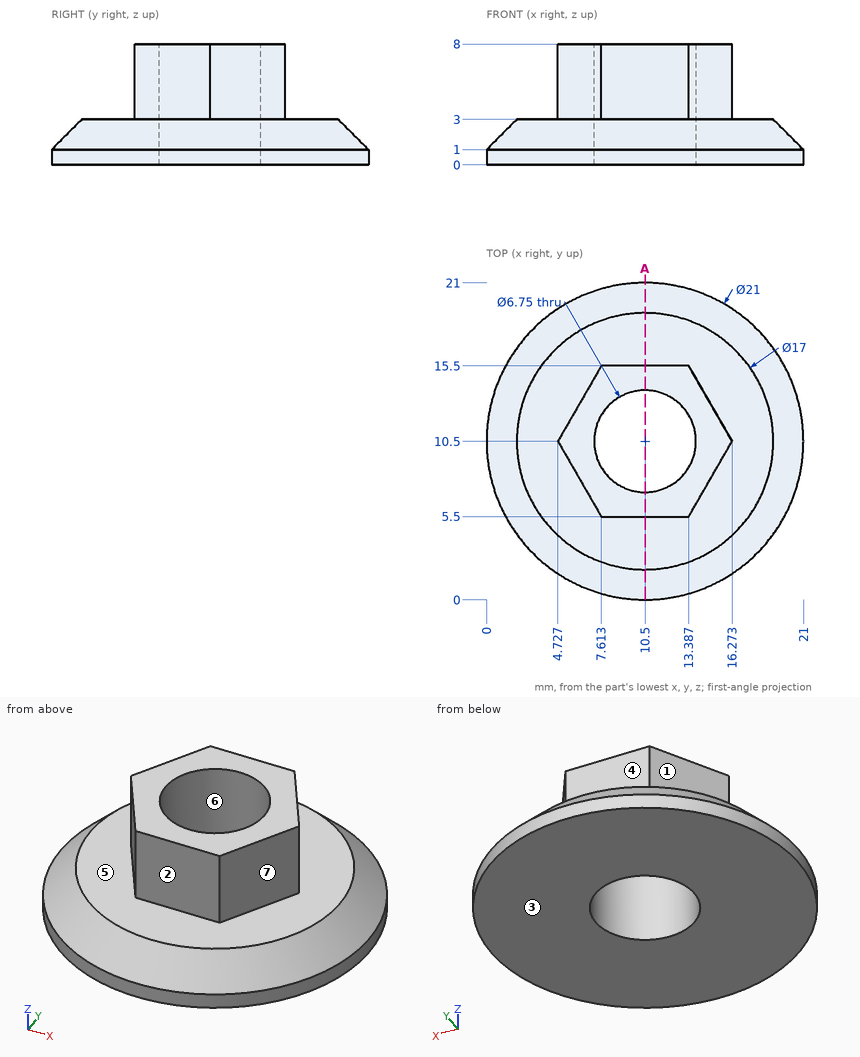
Geometry: see drawing. Coordinates: mm, zero at the bounding-box minimum. A direction names the side the tool comes from. Coordinates: 2 decimals unless noted, no trailing zeros. Loops run counter-clockwise (first coordinate to the right, second up) from the corner with the lowest first, then second, coordinate; pieces in that order, holes last.
(1) Material intervals for probe 1 along Y at (x, z) = (10.5, 5.75) (1 decimal); probe 2 along Z at (x, y) = (3.5, 7.5); probe 3 along Y at (x, z) = (7.75, 6.5) (1 decimal), sorted ascending.
(2) Set-up query: the marked faces 1, 2 and 3. Return all of +Z, -Z, +X, -X, +Y, -Y with unobstructed straight access to the full face (end or side cutting, diameter ignored); none if empty.
(3) Pull-direction query (Y, two-part tool) for the marked faces 4, 5, 6 and 7; classes: released by +Y, released by -Y, zero draft, split by the parting line, or undercut.
(4) Section A-A on x = 10.5. Return the cut outline in (y, z) (1 decimal).
(5) First-contact query: pin 1 Ø6 at (x, y) = (10.5, 10.5) entering from +Z; pin 2 Ø1.5 at (x, z) = (11.5, 2) entering from +Y (1 decimal); pin 3 Ø2 at (x, z) = (11, 4.5) entering from -Y; pin 4 Ø4 at (x, z) = (10.5, 4.5) entering from -Y. Flat tips, straight axial feed; report the tip coordinate or a pass-through.
Data:
1. probe 1: y = 5.5 to 7.1, 13.9 to 15.5
1. probe 2: z = 0 to 3
1. probe 3: y = 5.5 to 8.5, 12.5 to 15.5
2. face 1: +Z, -X, +Y
2. face 2: +Z, +X, -X, -Y
2. face 3: -Z, +X, -X, +Y, -Y
3. face 4: released by +Y
3. face 5: zero draft
3. face 6: undercut
3. face 7: released by -Y
4. outline: (0, 0) - (7.1, 0) - (7.1, 8) - (5.5, 8) - (5.5, 3) - (2, 3) - (0, 1) - close; (13.9, 0) - (21, 0) - (21, 1) - (19, 3) - (15.5, 3) - (15.5, 8) - (13.9, 8) - close
5. pin 1: passes through
5. pin 2: stops at y = 20.7
5. pin 3: stops at y = 5.5
5. pin 4: stops at y = 1.5
